Geometry: final body of the model. Coordinates: model frame, mm. Round coordinates to 2 decimals unless told otherwise and drop trailing zeros. Loops run counter-clockwise (first coordinate to the right, second up) from the corner with the lowest first, then second, coordinate; pieces in that order, holes last. Notation, with made-up numbers: (63.5, 13) - (81.5, 13) arc R34 ccw to (81.5, 49) - close; hole circle Ø11 at (2, 83.25). An arc over 180 degrees is marked (long way). Return JSON: item names as keys, results as strings. Group by question number.
1. Section B-B on z = -41. Return loops of the section in (x, y), and give its area (3 significant figures).
2. Material intervals for probe 1 along X at (y, z) = (-0.15, 66.5); probe 2 along Z at (x, y) = (5.25, 1); probe 3 along Y at (x, z) = (0.5, 22.5), sorted ascending.
3. First-contact query: pin 1 Ø8 at (y, z) = (-2, 20.5) entering from +X; pin 2 Ø0.8 at (x, y) = (4, 0) entering from +Z; pin 3 Ø2 at (x, z) = (0.5, 42.5) entering from -Y. Flat tips, straight axial feed; report the tip coordinate or a pass-through.
4. Section A-A on z = 5.5. Return loops of the section in (x, y), and give its area (3 significant figures).
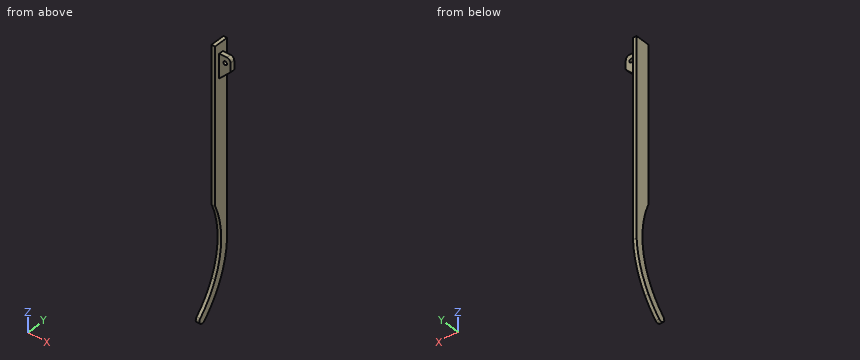
from build123d import *

# Parameters (mm, degrees)
SKETCH1_W           = 140
SKETCH1_H           = 8
BOSS_EXTRUDE1_DEPTH = 2
SKETCH3_W           = 7
SKETCH3_H           = 2.5
BOSS_EXTRUDE2_DEPTH = 6.3
SKETCH4_R           = 1
CUT_EXTRUDE1_DEPTH  = 4
SKETCH6_R           = 50
CUT_EXTRUDE3_DEPTH  = 14
BOSS_EXTRUDE4_DEPTH = 2
CUT_EXTRUDE5_DEPTH  = 2
FILLET6_R           = 2
FILLET7_R           = 2
SKETCH11_W          = 2
SKETCH11_H          = 8
BOSS_EXTRUDE5_DEPTH = 5.5
CHAMFER1_SIZE       = 6.3


with BuildPart() as part:
    # Sketch1 → Boss-Extrude1 (new body)
    with BuildSketch(Plane(origin=(0, 0, 0), x_dir=(0, 0, -1), z_dir=(1, 0, 0))):
        Rectangle(SKETCH1_W, SKETCH1_H)
    extrude(amount=BOSS_EXTRUDE1_DEPTH)

    # Sketch3 → Boss-Extrude2 (add)
    with BuildSketch(Plane(origin=(2, 0, 0), x_dir=(0, 0, -1), z_dir=(1, 0, 0))):
        with Locations((-66.5, 0)):
            Rectangle(SKETCH3_W, SKETCH3_H)
    extrude(amount=BOSS_EXTRUDE2_DEPTH)

    # Sketch4 → Cut-Extrude1 (cut)
    with BuildSketch(Plane(origin=(0, 1.25, 0), x_dir=(1, 0, 0), z_dir=(0, 1, 0))):
        with Locations(Location((5.3, -66.5, 0), (0, 0, 270))):
            Circle(SKETCH4_R)
    extrude(amount=-CUT_EXTRUDE1_DEPTH, mode=Mode.SUBTRACT)

    # Sketch6 → Cut-Extrude3 (cut)
    with BuildSketch(Plane(origin=(2, 0, 0), x_dir=(0, 0, -1), z_dir=(1, 0, 0))):
        with Locations((30, -49.921005204)):
            Circle(SKETCH6_R)
    extrude(amount=-CUT_EXTRUDE3_DEPTH, mode=Mode.SUBTRACT)

    # Sketch9 → Boss-Extrude4 (add)
    with BuildSketch(Plane(origin=(2, 0, 0), x_dir=(0, 0, -1), z_dir=(1, 0, 0))):
        with BuildLine():
            Line((69.093233498, -12.668903321), (66.197438424, -15.428318275))
            ThreePointArc((66.197438424, -15.428318275), (58.566223606, -8.884791089), (49.780325606, -4))
            Line((49.780325606, -4), (58.412343815, -4))
            ThreePointArc((58.412343815, -4), (64.029960524, -7.992950315), (69.093233498, -12.668903321))
        make_face()
    extrude(amount=-BOSS_EXTRUDE4_DEPTH)

    # Sketch10 → Cut-Extrude5 (cut)
    with BuildSketch(Plane(origin=(2, 0, 0), x_dir=(0, 0, -1), z_dir=(1, 0, 0))):
        with BuildLine():
            Line((30, 4.078994796), (98.693138082, 13.357457715))
            Line((98.693138082, 13.357457715), (83.74319787, -55.181108121))
            ThreePointArc((83.74319787, -55.181108121), (70.000284733, -13.644604869), (30, 4.078994796))
        make_face()
    extrude(amount=-CUT_EXTRUDE5_DEPTH, mode=Mode.SUBTRACT)

    # Fillet6
    fillet6_edges = [part.edges().sort_by_distance(p)[0] for p in [
        (1, -15.428318275, -66.197438424),
        (1, -12.668903321, -69.093233498),
    ]]
    fillet(fillet6_edges, radius=FILLET6_R - 0.0001)  # a hair under: the kernel refuses the full size

    # Fillet7
    fillet7_edges = [part.edges().sort_by_distance(p)[0] for p in [
        (8.3, 0, 70),
    ]]
    fillet(fillet7_edges, radius=FILLET7_R)

    # Sketch11 → Boss-Extrude5 (add)
    with BuildSketch(Plane.XY.offset(70)):
        with Locations((1, 0)):
            Rectangle(SKETCH11_W, SKETCH11_H)
    extrude(amount=BOSS_EXTRUDE5_DEPTH)

    # Chamfer1
    chamfer1_edges = [part.edges().sort_by_distance(p)[0] for p in [
        (2, 0, 63),
    ]]
    chamfer(chamfer1_edges, length=CHAMFER1_SIZE - 0.0001)  # a hair under: the kernel refuses the full size


solid = part.part
Taken from the geometry:
{
 "1": {"outline": "(0, -1.15) - (2, -1.15) - (2, 2.95) - (0, 2.95) - close", "area": "8.19 mm2"},
 "2": {"probe 1": "0 to 4.3, 6.3 to 8.3", "probe 2": "59.95 to 65.5, 67.5 to 70", "probe 3": "-4 to 4"},
 "3": {"pin 1": "x = 2", "pin 2": "z = 70", "pin 3": "y = -4"},
 "4": {"outline": "(0, -4) - (2, -4) - (2, 4) - (0, 4) - close", "area": "16.0 mm2"}
}
